Design review of the part built by this model. Coordinates are the model's own, in mm. A direction names the side the tool comes from. Give positions to 0.01 mm unless a question says otherwise; leave off trailing zeros. Write each loop counter-clockwise with the first axis right and the second up, starting at its lowest first coordinate (ties: lowest second). Pieces come first, ordered by that corner, then holes. Notation, with made-up numbers: (-22, 66.25) -> (23, 66.25) arc R28 ccw to (23, 92.25) -> close; hole circle Ø8 at (78.25, 62). An arc over 180 degrees is marked (long way). Use CSV: the item, a comma, the result in double quotes.
```python
from build123d import *


with BuildPart() as f1:
    # F0 (on Front) → F1 (revolve)
    with BuildSketch(Plane.XZ):
        Polygon((5, 0), (2.5, 0), (2.5, -7.5), (0, -7.5), (0, -32), (0, -35), (0, -50), (3.5, -50), (5, -50), (5, -35), (6, -35), (6, -32), (5, -32), align=None)
        Polygon((3.5, -50), (0, -50), (0, -55), (3.5, -55), (5, -50), align=None)
    revolve(axis=Axis((0, 0, -28.75), (0, 0, -1)))


solid = f1.part
```
(1) For line 1 along Y through (x, z) = (0, -5.5); line 2 along Z through (x, y) = (-3.5, -3.75), list the stretches that pass through material, from the lowest coordinate up. Write a range as [from, to].
Established:
line 1,"y = [-5, -2.5], [2.5, 5]"
line 2,"z = [-35, -32]"
(2) Mouldability with a two-part tool opening along Y and no side actions: class faces 1 (the face through (-6, 0, -33)), 2 (the face through (-4, -4, -32)), 3 (the face through (0, 0, -7.5)) as +Y half, -Y half, draft (parallel to the pull), parting line (faces both ways), or undercut.
Established:
face 1,"parting line"
face 2,"draft"
face 3,"undercut"
(3) Take a section at C-C (z = -42). Write out the cut boundary in (x, y).
Established:
outline,"circle Ø10 at (0, 0)"
(4) Tool access review of faces 4 (the face through (2, 2, 0)), 5 (the face through (-0.54, 2.44, -3.8)), 6 (the face through (4, -4, -35)): name each direction out of +Z, -Z, +X, -X, +Y, -Y from which nothing blocks a thin tool from reaching the whole face with its end or side.
Established:
face 4,"+Z, +X, -X, +Y, -Y"
face 5,"+Z"
face 6,"-Z"
(5) Clearance check with flat-ended pins moving along their axes: pin 1 (5.5 mm diameter, centred on x = 1, y = 0, fed in from +Z); pin 2 (6 mm diameter, centred on x = -4.5, z = -28.5, fed in from -Y); pin 3 (1.5 mm diameter, centred on x = 0, z = -19.5, fed in from -Y); pin 4 (5 mm diameter, centred on y = -2.5, z = -41.5, fed in from +X). State where each tip first meets the part, or that it passes through.
Established:
pin 1,"stops at z = 0"
pin 2,"stops at y = -4.77"
pin 3,"stops at y = -5"
pin 4,"stops at x = 5"
(6) Take a section at A-A (x = 0). Write out the cut boundary in (y, z).
Established:
outline,"(-6, -35) -> (-5, -35) -> (-5, -50) -> (-3.5, -55) -> (3.5, -55) -> (5, -50) -> (5, -35) -> (6, -35) -> (6, -32) -> (5, -32) -> (5, 0) -> (2.5, 0) -> (2.5, -7.5) -> (-2.5, -7.5) -> (-2.5, 0) -> (-5, 0) -> (-5, -32) -> (-6, -32) -> close"
